Autodesk Inventor part; units mm, degrees
ref_plane "YZ Plane" through (0, 0, 0) normal (1, 0, 0) x (0, 1, 0)
ref_plane "XZ Plane" through (0, 0, 0) normal (0, 1, 0) x (-1, 0, 0)
ref_plane "XY Plane" through (0, 0, 0) normal (0, 0, 1) x (1, 0, 0)
sketch "Sketch1" plane through (0, 0, 0) normal (0, 1, 0) x (-1, 0, 0)
  line L0 (59.8, 32.5) -> (-59.8, 32.5)
  line L1 (-59.8, 32.5) -> (-59.8, -32.5)
  line L2 (-59.8, -32.5) -> (59.8, -32.5)
  line L3 (59.8, -32.5) -> (59.8, 32.5)
  line L4 (59.8, 32.5) -> (-59.8, -32.5) construction
  line L5 (-59.8, 32.5) -> (59.8, -32.5) construction
  point P0 (0, 0)
  dimension "d0" = 119.6
  dimension "d1" = 65
extrude "Extrusion1" add sketch "Sketch1" along normal blind 1.5
sketch "Sketch2" plane through (0, 1.5, 0) normal (0, 1, 0) x (1, 0, 0)
  line L0 (59.8, -32.5) -> (59.8, 32.5)
  line L1 (-59.8, -29.75) -> (59.8, -29.75)
  line L2 (59.8, -29.75) -> (59.8, 29.75)
  line L3 (59.8, 29.75) -> (-59.8, 29.75)
  line L4 (-59.8, 29.75) -> (-59.8, -29.75)
  line L5 (-59.8, -29.75) -> (59.8, 29.75) construction
  line L6 (59.8, -29.75) -> (-59.8, 29.75) construction
  line L7 (59.8, 29.75) -> (56.3, 29.75)
  line L8 (56.3, 29.75) -> (56.3, 30.25)
  line L9 (56.3, 30.25) -> (59.8, 30.25)
  line L10 (59.8, 30.25) -> (59.8, 29.75)
  line L11 (56.3, 29.75) -> (56.3, 29.25)
  line L12 (56.3, 29.25) -> (59.8, 29.25)
  line L13 (59.8, 29.25) -> (59.8, 29.75)
  line L14 (0, 0) -> (0, 29.75)
  line L15 (0, 0) -> (37, 0)
  line L16 (-59.8, 29.75) -> (-56.3, 29.75)
  line L17 (-56.3, 29.75) -> (-56.3, 30.25)
  line L18 (-56.3, 30.25) -> (-59.8, 30.25)
  line L19 (-59.8, 30.25) -> (-59.8, 29.75)
  line L20 (-56.3, 29.75) -> (-56.3, 29.25)
  line L21 (-56.3, 29.25) -> (-59.8, 29.25)
  line L22 (-59.8, 29.25) -> (-59.8, 29.75)
  line L23 (59.8, -29.75) -> (56.3, -29.75)
  line L24 (56.3, -29.75) -> (56.3, -30.25)
  line L25 (56.3, -30.25) -> (59.8, -30.25)
  line L26 (59.8, -30.25) -> (59.8, -29.75)
  line L27 (56.3, -29.75) -> (56.3, -29.25)
  line L28 (56.3, -29.25) -> (59.8, -29.25)
  line L29 (59.8, -29.25) -> (59.8, -29.75)
  line L30 (-59.8, -29.75) -> (-56.3, -29.75)
  line L31 (-56.3, -29.75) -> (-56.3, -30.25)
  line L32 (-59.8, -30.25) -> (-59.8, -29.75)
  line L33 (-56.3, -29.75) -> (-56.3, -29.25)
  line L34 (-56.3, -29.25) -> (-59.8, -29.25)
  line L35 (-59.8, -29.25) -> (-59.8, -29.75)
  line L36 (-56.3, -30.25) -> (-59.8, -30.25)
  dimension "d4" = 59.5
  dimension "d5" = 3.5
  dimension "d6" = 0.5
extrude "Extrusion2" add sketch "Sketch2" along normal blind 3.5 contours L25 L24 L1 L0 | L1 L27 L28 L0 | L12 L11 L3 L0 | L31 L36 L32 L1 | L1 L4 L34 L33 | L3 L8 L9 L0 | L4 L3 L20 L21 | L3 L19 L18 L17
hole "Hole1" at (-58.05, 3.25, 30.25) direction (0, 0, -1) diameter 3 end through all
hole "Hole2" at (58.05, 3.25, 30.25) direction (0, 0, -1) diameter 3 end through all
properties part number "Bumper big"
Source: CAD feature listing. Evaluate the final solid. Frame: model axes, mm. Round coordinates to 2 decimals unless told otherwise and drop trailing zeros. Write each loop counter-clockwise with the first axis right and the second up, starting at its lowest first coordinate (ties: lowest second). Pieces come first, ordered by that corner, then holes. Notation, with made-up numbers: M 25,76.25 L 54,76.25 A18 cw 54,90.25 Z; hole C 31,9.25 d1. An arc over 180 degrees is marked long. One line per item, written item: value. Start each with the question number.
Item 1: Pin query (flat end, axial travel): pin 1 (1.8 mm diameter, centred on x = 57, y = 3, fed in from +Z); pin 2 (3 mm diameter, centred on x = 57.5, y = 4, fed in from -Z); pin 3 (1 mm diameter, centred on x = 33, y = 3, fed in from -Z); pin 4 (3 mm diameter, centred on x = -44.5, z = -21.5, fed in from +Y). Return the tip coordinate at first contact, or that it passes through.
Item 2: Ray query, L1, parallel to X at y = 3.25, z = 29.9; L2, parallel to Y at x = -58.05, z = 30.05; L3, parallel to Y at x = 40, z = 17. Return the intervals inside material, ascending. Write a range as from..to.
Item 3: Section query B-B (x = -58.05). Return the cut outline in (y, z), plus the area to 3 significant figures.
Item 4: Section query A-A (y = 3.25). State how many separate pieces and enclosed holes the cut face has, plus the area to 3 significant figures.
Item 5: Section query C-C (x = -12). Return the cut outline in (y, z), plus the area to 3 significant figures.
Item 6: Section query D-D (z = -13). Return the cut outline in (x, y).
Item 7: Mould query, pull axis X, two halves, no side actions, for faces 1 (the cylindrical face through (-56.586, 3.575, -29.757)), 2 (the flat face through (59.8, 1, 8)), 3 (the flat face through (-59.8, 1, -8)), 4 (the flat face through (1, 0, 0)). Classes: pulls with the +X half, pulls with the -X half, needs draft (parallel to the pull), parting line crosses it, or undercut.
Result set:
1. pin 1: stops at z = 30.25
1. pin 2: stops at z = -30.25
1. pin 3: passes through
1. pin 4: stops at y = 1.5
2. L1: x = -59.8..-59.55, -56.55..-56.3, 56.3..56.55, 59.55..59.8
2. L2: y = 0..1.75, 4.75..5
2. L3: y = 0..1.5
3. outline: M 0,-32.5 L 1.5,-32.5 L 1.5,-30.25 L 1.75,-30.25 L 1.75,-29.25 L 1.5,-29.25 L 1.5,29.25 L 1.75,29.25 L 1.75,30.25 L 1.5,30.25 L 1.5,32.5 L 0,32.5 Z; M 4.75,-30.25 L 5,-30.25 L 5,-29.25 L 4.75,-29.25 Z; M 4.75,29.25 L 5,29.25 L 5,30.25 L 4.75,30.25 Z
3. area: 98.5 mm²
4. separate pieces: 8
4. enclosed holes: 0
4. area: 2.00 mm²
5. outline: M 0,-32.5 L 1.5,-32.5 L 1.5,32.5 L 0,32.5 Z
5. area: 97.5 mm²
6. outline: M -59.8,0 L 59.8,0 L 59.8,1.5 L -59.8,1.5 Z
7. face 1: undercut
7. face 2: pulls with the +X half
7. face 3: pulls with the -X half
7. face 4: needs draft
